Autodesk Inventor part; units mm, degrees
ref_plane "YZ Plane" through (0, 0, 0) normal (1, 0, 0) x (0, 1, 0)
ref_plane "XZ Plane" through (0, 0, 0) normal (0, 1, 0) x (-1, 0, 0)
ref_plane "XY Plane" through (0, 0, 0) normal (0, 0, 1) x (1, 0, 0)
sketch "Sketch1" plane through (0, 0, 0) normal (0, 0, 1) x (1, 0, 0)
  line L0 (0, 0) -> (7.62, 0)
  line L1 (7.62, 0) -> (7.62, 5.08)
  line L2 (7.62, 5.08) -> (0, 5.08)
  line L3 (0, 5.08) -> (0, 0)
  dimension "d0" = 7.62
  dimension "d1" = 5.08
extrude "Extrusion1" add sketch "Sketch1" along normal blind 259.8166
sketch "Sketch2" plane through (0, 0, 259.8166) normal (0, 0, 1) x (1, 0, 0)
  circle A0 centre (3.8115, 2.54) radius 5.08
  line L0 (7.62, 5.08) -> (0, 5.08)
  line L1 (7.62, 0) -> (7.62, 5.08)
  point P0 (0, 0)
  dimension "d4" = 10.16
  dimension "d5" = 2.54
  dimension "d6" = 3.8085
extrude "Extrusion2" add sketch "Sketch2" along normal blind 12.7
sketch "Sketch3" plane through (0, 0, 0) normal (0, 0, -1) x (-1, 0, 0)
  circle A0 centre (-3.8115, 2.54) radius 5.08
  circle A1 centre (-3.8115, 2.54) radius 5.08
  point P0 (0, 0)
  dimension "d9" = 10.16
extrude "Extrusion3" add sketch "Sketch3" along normal blind 12.7
sketch "Sketch4" plane through (3.8115, 2.54, -12.7) normal (0, 0, -1) x (-1, 0, 0)
  circle A0 centre (0, 0) radius 7.62
  point P0 (3.8115, -2.54)
  dimension "d12" = 15.24
extrude "Extrusion4" add sketch "Sketch4" along normal blind 3.175
sketch "Sketch5" plane through (0, 5.08, 259.8166) normal (0, 1, 0) x (1, 0, 0)
  line L0 (7.62, 259.8166) -> (7.62, 0)
  line L1 (-1.2685, 259.8166) -> (8.8915, 259.8166)
  circle A0 centre (4.445, 129.9083) radius 20
  point P0 (0, 259.8166)
  dimension "d15" = 3.175
  dimension "d16" = 259.8166
  dimension "d17" = 129.9083
  dimension "d18" = 40
extrude "Extrusion5" add sketch "Sketch5" against normal up to surface (5.08 mm away)
sketch "Sketch6" plane through (0, 5.08, 259.8166) normal (0, 1, 0) x (1, 0, 0)
  circle A0 centre (4.445, 129.9083) radius 20
  arc A1 (0, 149.4081) -> (0, 110.4085) centre (4.445, 129.9083) ccw
  circle A2 centre (4.445, 129.9083) radius 12.5
  point P0 (0, 259.8166)
  point P1 (-8.055, 129.9083)
  point P2 (4.445, 142.4083)
  point P3 (16.945, 129.9083)
  point P4 (4.445, 117.4083)
  dimension "d21" = 40
  dimension "d22" = 0
  dimension "d23" = 0
  dimension "d24" = 25
hole "Hole1" at (4.445, 5.08, 129.9083) at (-8.055, 5.08, 129.9083) at (4.445, 5.08, 117.4083) at (16.945, 5.08, 129.9083) at (4.445, 5.08, 142.4083) direction (0, -1, 0) diameter 4 end through all
properties part number "MotorMount_Part"
Source: CAD feature listing. Evaluate the final solid. Frame: model axes, mm. A direction names the side the tool comes from. Give positions to 0.01 mm unless a question says otherwise; leave off trailing zeros. Write each loop counter-clockwise with the first axis right and the second up, starting at its lowest first coordinate (ties: lowest second). Pieces come first, ordered by that corner, then holes.
1. Access query for faces 4 (the face through (0, 3, 54)), 5 (the face through (1, 0, 129)), 6 (the face through (-1.034, 1.014, -6.261)), 7 (the face through (7.62, 3, 54)). Directions: +Z, -Z, +X, -X, +Y, -Y. A direction counts if a zero-diameter tool reaches every point of the face in a straight line with its end or side. Return the directions, or none.
2. Section query B-B (z = 199.5). Return the cut outline in (x, y), then the cut area to 3 significant figures.
3. First-contact query: pin 1 (1.5 mm diameter, centred on y = 6.5, z = 29, fed in from +X); pin 2 (8 mm diameter, centred on y = 6.5, z = 217.5, fed in from +X); pin 3 (4 mm diameter, centred on y = 3.5, z = 62, fed in from -X); pin 4 (1.5 mm diameter, centred on x = 14.5, y = 4.5, fed in from +Z). Flat tips, straight axial feed; report the tip coordinate or a pass-through.
4. Material intervals for line 1 along Z through (x, y) = (4, 6.75) (3 decimals); line 2 along Z through (x, y) = (9, 2) (3 decimals); line 3 along Y through (x, z) = (12, 134.5), sorted ascending.
5. Section query A-A (y = 2.54). Return the cut outline in (x, z) (1 decimal).
6. Pull-direction query (Z, two-part tool) for faces 1 (the face through (4, 3, -15.875)), 2 (the face through (0, 5.08, 129)), 3 (the face through (-0.22, 5.63, 266.08)); classes: +Z half, -Z half, draft (parallel to the pull), parting line (faces both ways), or undercut.
Output values:
1. face 4: -X, +Y, -Y
1. face 5: +X, -X, -Y
1. face 6: none
1. face 7: +X, +Y, -Y
2. outline: (0, 0) - (7.62, 0) - (7.62, 5.08) - (0, 5.08) - close
2. area: 38.7 mm2
3. pin 1: passes through
3. pin 2: stops at x = 7.62
3. pin 3: stops at x = 0
3. pin 4: stops at z = 147.61
4. line 1: z = -15.875 to 0, 259.817 to 272.517
4. line 2: z = -15.875 to -12.7, 110.434 to 149.383
4. line 3: y = 0 to 5.08
5. outline: (-3.8, -15.9) - (11.4, -15.9) - (11.4, -12.7) - (8.9, -12.7) - (8.9, 0) - (7.6, 0) - (7.6, 110.2) arc R20 ccw to (7.6, 149.7) - (7.6, 259.8) - (8.9, 259.8) - (8.9, 272.5) - (-1.3, 272.5) - (-1.3, 259.8) - (0, 259.8) - (0, 149.4) arc R20 ccw to (0, 110.4) - (0, 0) - (-1.3, 0) - (-1.3, -12.7) - (-3.8, -12.7) - close; hole circle Ø4 at (-8.1, 129.9); hole circle Ø4 at (4.4, 117.4); hole circle Ø4 at (4.4, 129.9); hole circle Ø4 at (4.4, 142.4); hole circle Ø4 at (16.9, 129.9)
6. face 1: -Z half
6. face 2: undercut
6. face 3: draft
